Here's how the part is built. I have some questions about the finished solid (model axes, mm). Face numbers are marked on the shaded views. A direction names the side the tool comes from. Give positions to 0.01 mm unless a question says otherwise; leave off trailing zeros. Order: outer loops, then holes, each group sorted by start corner. A loop starts at its lowest first (then second) coordinate and runs counter-clockwise, first axis right, second up.
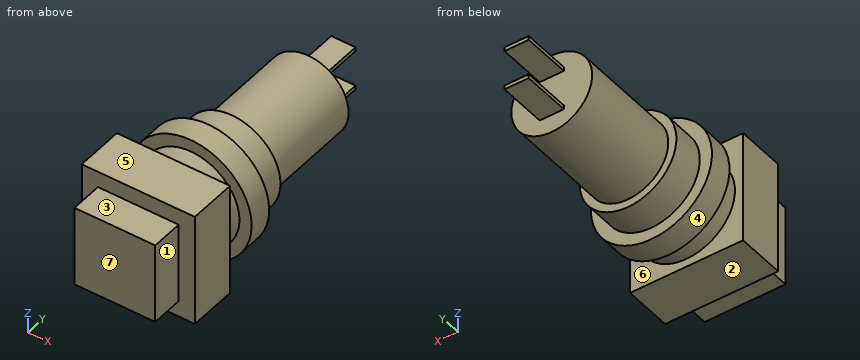
from build123d import *

# Parameters (mm, degrees)
SKETCH1_W           = 10
SKETCH1_H           = 10
BOSS_EXTRUDE1_DEPTH = 4
SKETCH2_W           = 14
SKETCH2_H           = 14
BOSS_EXTRUDE2_DEPTH = 6
SKETCH3_R           = 6
BOSS_EXTRUDE3_DEPTH = 3
SKETCH4_R           = 7.5
BOSS_EXTRUDE4_DEPTH = 3
SKETCH5_R           = 6
BOSS_EXTRUDE5_DEPTH = 4
SKETCH6_R           = 5
BOSS_EXTRUDE6_DEPTH = 13
SKETCH7_W           = 3
SKETCH7_H           = 0.5
BOSS_EXTRUDE7_DEPTH = 6


with BuildPart() as part:
    # Sketch1 → Boss-Extrude1 (new body)
    with BuildSketch(Plane(origin=(0, 0, 0), x_dir=(1, 0, 0), z_dir=(0, 1, 0))):
        Rectangle(SKETCH1_W, SKETCH1_H)
    extrude(amount=BOSS_EXTRUDE1_DEPTH)

    # Sketch2 → Boss-Extrude2 (add)
    with BuildSketch(Plane(origin=(0, 4, 0), x_dir=(1, 0, 0), z_dir=(0, 1, 0))):
        Rectangle(SKETCH2_W, SKETCH2_H)
    extrude(amount=BOSS_EXTRUDE2_DEPTH)

    # Sketch3 → Boss-Extrude3 (add)
    with BuildSketch(Plane(origin=(0, 10, 0), x_dir=(1, 0, 0), z_dir=(0, 1, 0))):
        Circle(SKETCH3_R)
    extrude(amount=BOSS_EXTRUDE3_DEPTH)

    # Sketch4 → Boss-Extrude4 (add)
    with BuildSketch(Plane(origin=(0, 13, 0), x_dir=(1, 0, 0), z_dir=(0, 1, 0))):
        Circle(SKETCH4_R)
    extrude(amount=BOSS_EXTRUDE4_DEPTH)

    # Sketch5 → Boss-Extrude5 (add)
    with BuildSketch(Plane(origin=(0, 16, 0), x_dir=(1, 0, 0), z_dir=(0, 1, 0))):
        Circle(SKETCH5_R)
    extrude(amount=BOSS_EXTRUDE5_DEPTH)

    # Sketch6 → Boss-Extrude6 (add)
    with BuildSketch(Plane(origin=(0, 20, 0), x_dir=(1, 0, 0), z_dir=(0, 1, 0))):
        Circle(SKETCH6_R)
    extrude(amount=BOSS_EXTRUDE6_DEPTH)

    # Sketch7 → Boss-Extrude7 (add)
    with BuildSketch(Plane(origin=(0, 33, 0), x_dir=(1, 0, 0), z_dir=(0, 1, 0))):
        with Locations((0, -2.5)):
            Rectangle(SKETCH7_W, SKETCH7_H)
        with Locations((0, 2.5)):
            Rectangle(SKETCH7_W, SKETCH7_H)
    extrude(amount=BOSS_EXTRUDE7_DEPTH)


solid = part.part
Q1. I need wall thicknesses on L1, parallel to Y at x = -6.75, z = 2; L2, parallel to Y at x = -0.25, z = -4; L3, parallel to Y at x = -4, z = -4. Which ranges of each line are inside material? Lowest first, please.
Filled sheet:
L1: y = 4 to 10, 13 to 16
L2: y = 0 to 33
L3: y = 0 to 20
Q2. If we section it at A-A on y = 34.5: List the corners of the cut face in (x, z) for me, plus the area to 3 significant figures.
Filled sheet:
outline: (-1.5, -2.75) - (1.5, -2.75) - (1.5, -2.25) - (-1.5, -2.25) - close; (-1.5, 2.25) - (1.5, 2.25) - (1.5, 2.75) - (-1.5, 2.75) - close
area: 3.00 mm2
Q3. If we section it at D-D on z = 6.5: List the corners of the cut face in (x, y) for me, plus the area to 3 significant figures.
Filled sheet:
outline: (-7, 4) - (7, 4) - (7, 10) - (-7, 10) - close; (-3.74, 13) - (3.74, 13) - (3.74, 16) - (-3.74, 16) - close
area: 106 mm2
Q4. For the marked faces 1, 2, 3 and 4, which set-ups out of +Z, -Z, +X, -X, +Y, -Y let a thin tool reach every point of the face, with its end or its side?
Filled sheet:
face 1: +Z, -Z, +X, -Y
face 2: -Z, +X, -X, -Y
face 3: +Z, +X, -X, -Y
face 4: +Y
Q5. I'm going to push flat-ended pins straight in: P1, Ø3, axis at x = -5, z = 3.5, coming from the -Y side; P2, Ø0.9, axis at x = -0.5, y = 36, coming from the +Z side; P3, Ø2, axis at x = -1.5, y = 1.5, coming from the +Z side; P4, Ø6, axis at y = 11, z = 4, coming from the +X side. Where does each tip first touch, or does it pass through?
Filled sheet:
P1: stops at y = 0
P2: stops at z = 2.75
P3: stops at z = 5
P4: stops at x = 7.29
Q6. If we section it at B-B on z = 0: List the corners of the cut face in (x, y) for me, plus the area to 3 significant figures.
Filled sheet:
outline: (-7.5, 13) - (-6, 13) - (-6, 10) - (-7, 10) - (-7, 4) - (-5, 4) - (-5, 0) - (5, 0) - (5, 4) - (7, 4) - (7, 10) - (6, 10) - (6, 13) - (7.5, 13) - (7.5, 16) - (6, 16) - (6, 20) - (5, 20) - (5, 33) - (-5, 33) - (-5, 20) - (-6, 20) - (-6, 16) - (-7.5, 16) - close
area: 383 mm2
Q7. Thinking about a two-plate mould opening in Y: for the marked faces 5, 6 and 7, which applies, released by +Y, released by -Y, zero draft, split by the parting line, or undercut?
Filled sheet:
face 5: zero draft
face 6: undercut
face 7: released by -Y
Q8. If we section it at C-C on x = -3.5: List the corners of the cut face in (y, z) for me, plus the area to 3 significant figures.
Filled sheet:
outline: (0, -5) - (4, -5) - (4, -7) - (10, -7) - (10, -4.87) - (13, -4.87) - (13, -6.63) - (16, -6.63) - (16, -4.87) - (20, -4.87) - (20, -3.57) - (33, -3.57) - (33, 3.57) - (20, 3.57) - (20, 4.87) - (16, 4.87) - (16, 6.63) - (13, 6.63) - (13, 4.87) - (10, 4.87) - (10, 7) - (4, 7) - (4, 5) - (0, 5) - close
area: 325 mm2
